Autodesk Inventor part; units mm, degrees
ref_plane "YZ Plane" through (0, 0, 0) normal (1, 0, 0) x (0, 1, 0)
ref_plane "XY Plane" through (0, 0, 0) normal (0, 0, 1) x (1, 0, 0)
ref_plane "UCS1: YZ Plane" through (0, 0, 0) normal (1, 0, 0) x (0, 1, 0)
sketch "Sketch2" plane through (0, 0, 0) normal (1, 0, 0) x (0, 1, 0)
  circle A0 centre (0, -60) radius 27.5
  line L0 (27.5, -162.5) -> (-27.5, -162.5)
  line L1 (0, -60) -> (0, -162.5) construction
  line L2 (-27.5, -60) -> (-27.5, -162.5)
  line L3 (27.5, -60) -> (27.5, -162.5)
  circle A1 centre (0, 0) radius 30.5
  line L4 (-30.4619, -1.525) -> (-27.4656, -61.375)
  line L5 (30.4619, -1.525) -> (27.4656, -61.375)
  line L6 (30.5382, 0) -> (-30.5382, 0)
  point P0 (-30.5, 0)
  point P1 (30.5, 0)
  point P2 (-30.5, 0)
  point P3 (-27.5, -60.6879)
  point P4 (27.5, -60.6879)
  dimension "d1" = 55
  dimension "d3" = 55
  dimension "d26" = 61
  dimension "d33" = 60
  dimension "d39" = 162.5
extrude "Extrusion1" add sketch "Sketch2" along normal mid plane 50 contours A0
extrude "Extrusion2" add sketch "Sketch2" against normal blind 50 from surface at 25 contours L3 L5 A0 | A0 L4 L2 | L5 L3 L0 L2 L4 A0
sketch "Sketch5" plane through (25, -27.5, -162.5) normal (0, 0, -1) x (-1, 0, 0)
  circle A0 centre (25, 27.5) radius 10
  line L0 (50, 55) -> (50, 0)
  line L1 (50, 55) -> (0, 55)
  point P0 (25, 27.5)
  point P1 (50, 27.5)
  point P2 (-45, 0)
  point P3 (25, 55)
  dimension "d22" = 20
extrude "Extrusion4" cut sketch "Sketch5" against normal blind 60
ref_plane "Work Plane1" through (0, 0, -60) normal (-1, 0, 0) x (0, 0, -1)
sketch "Sketch4" plane through (0, 0, -60) normal (-1, 0, 0) x (0, 0, -1)
  circle A0 centre (-60, 0) radius 162.5
  line L0 (102.5, -27.5) -> (102.5, 27.5)
  line L1 (-222.5, 0) -> (102.5, 0)
  line L2 (102.5, 0) -> (102.5, 27.5)
  line L3 (102.5, 27.5) -> (0, 27.5)
  line L4 (102.5, 27.5) -> (102.5, 40.4047)
  line L5 (102.5, 40.4047) -> (97.3967, 40.4047)
  point P0 (100.1562, 27.5)
  point P1 (102.5, 0)
revolve "Revolution1" cut sketch "Sketch4" angle 360 about axis through (0, 0, 162.5) along (0, 0, -1) contours L5 L4 L3 A0 | L3 L0 A0
extrude "Extrusion5" add sketch "Sketch2" along normal mid plane 50 contours A0 L2 L4 A1 L5 L3 | A1 L6 | L6 A1
properties part number "shank_inventor"
Input: part model. Units: mm. Frame: model coordinates. A direction names the side the tool comes from. Round coordinates to 2 decimals unless told otherwise and drop trailing zeros. Write each loop counter-clockwise with the first axis right and the second up, starting at its lowest first coordinate (ties: lowest second). Pieces come first, ordered by that corner, then holes. Notation, with made-up numbers: (82.25, -7) -> (105.25, -7) arc R23 cw to (105.25, 16) -> close; hole circle Ø5 at (38, -12.5). An arc over 180 degrees is marked (long way). Answer as CSV lines item,"result".
1. Section B-B (y = 0). Return the cut outline in (x, z), plus the area to 3 significant figures.
Geometry says:
outline,"(-25, -160.57) arc R162.5 ccw to (-10, -162.19) -> (-10, -102.5) -> (10, -102.5) -> (10, -162.19) arc R162.5 ccw to (25, -160.57) -> (25, 30.5) -> (-25, 30.5) -> close"
area,"8,420 mm^2"
2. Section D-D (z = 16.5). Return the cut outline in (x, y), plus the area to 3 significant figures.
Geometry says:
outline,"(-25, -25.65) -> (25, -25.65) -> (25, 25.65) -> (-25, 25.65) -> close"
area,"2,570 mm^2"
3. Section A-A (z = -140). Return the cut outline in (x, y).
Geometry says:
outline,"(-25, -27.5) -> (25, -27.5) -> (25, 27.5) -> (-25, 27.5) -> close; hole circle Ø20 at (0, 0)"
4. Contact query for flat-ended pins moving along their axis: P1, Ø8, axis at x = -2.5, y = 7.5, coming from the +Z side; P2, Ø2, axis at x = -1.5, z = -114, coming from the +Y side; P3, Ø15, axis at x = -1.5, z = -90, coming from the -Y side. Output: stop coordinate, or through.
Geometry says:
P1,"stops at z = 30.3"
P2,"stops at y = 27.5"
P3,"stops at y = -27.5"
5. Section C-C (x = -5). Return the cut outline in (y, z) (3 decimals), plus the area to 3 significant figures.
Geometry says:
outline,"(-30.462, -1.525) -> (-27.5, -60.688) -> (-27.5, -160.078) arc R162.423 ccw to (-8.66, -162.192) -> (-8.66, -102.5) -> (8.66, -102.5) -> (8.66, -162.192) arc R162.423 ccw to (27.5, -160.078) -> (27.5, -60.688) -> (30.462, -1.525) arc R30.5 ccw (long way) to start"
area,"9,500 mm^2"
6. Reachability of faces 1 (the flat face through (25, 0, -64)), 2 (the flat face through (0, 27.5, -110)), 3 (the flat face through (0, -27.5, -110)), 4 (the flat face through (0, 0, -102.5)) from +Z, -Z, +X, -X, +Y, -Y: full face, straight path, thin tool, end or side. Return the list, or none.
Geometry says:
face 1,"+Z, -Z, +X, +Y, -Y"
face 2,"-Z, +X, -X, +Y"
face 3,"-Z, +X, -X, -Y"
face 4,"-Z"
7. Mould query, pull axis Y, two halves, no side actions, for faces 5 (the flat face through (-25, 0, -64)), 6 (the flat face through (-0.4, 29, -30.7)), 7 (the cylindrical face through (2.17, -9.76, -132.76)). Classes: +Y half, -Y half, draft (parallel to the pull), parting line (faces both ways), or undercut.
Geometry says:
face 5,"draft"
face 6,"+Y half"
face 7,"undercut"
8. Ray query, L1, parallel to X at y = 0, z = -138; L2, parallel to Y at x = 0, z = -122; L3, parallel to Y at x = 7, z = 0.5. Return the intervals inside material, ascending. Write a range as [from, to].
Geometry says:
L1,"x = [-25, -10], [10, 25]"
L2,"y = [-27.5, -10], [10, 27.5]"
L3,"y = [-30.5, 30.5]"
